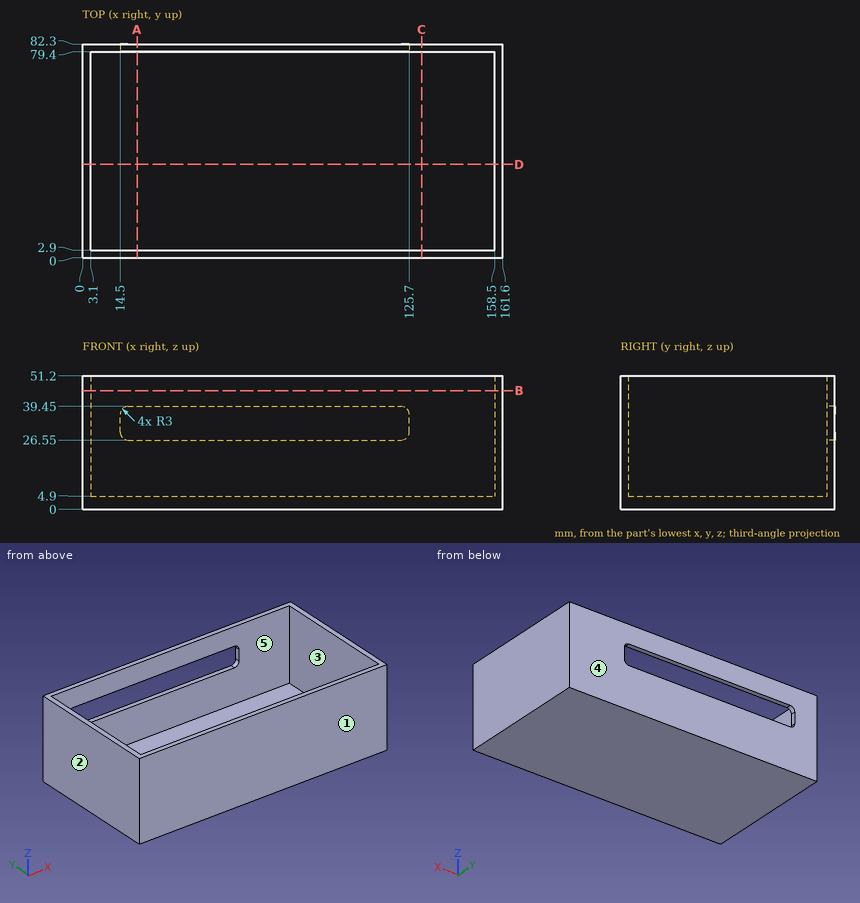
The figure shows three views and two pictorial views of one solid part (mm, origin at its lowest corner). Answer the questions. A direction names the side the tool comes from. Coordinates: 2 decimals unless noted, no trailing zeros. Order: outer loops, then holes, each group sorted by start corner. A loop starts at its lowest first (then second) coordinate and runs counter-clockwise, first axis right, second up.
Q1. Given P1, Ø8, axis at x = 45, y = 58.5, coming from the +Z side, flat-ended and moving along its own axis, determine where the tip first touches the part or whether it passes through.
Q2. A cutting plane is placed at A-A, the plane x = 21. Write down the section's boundary in (y, z).
Q3. A cutting plane is placed at C-C, the plane x = 130.5. Write down the section's boundary in (y, z), and give its area (3 significant figures).
Q4. A cutting plane is placed at D-D, the plane y = 36. Write down the section's boundary in (x, z), and give its area (3 significant figures).
Q5. For a pull along X with two mould halves and no side action, classify the marked faces 1, 2 and 3 as pulls with the +X half, pulls with the -X half, needs draft (parallel to the pull), parting line crosses it, or undercut.
Q6. Consider line 1 (Y direction, x = 85.5, z = 39.5); line 2 (X direction, y = 30.5, z = 28); line 3 (Z direction, x = 50, y = 66.5). Determine where each line is inside the solid, lowest interval first.
Q7. A cutting plane is placed at B-B, the plane z = 45.5. Write down the section's boundary in (x, y).
Q8. Which of the six approach directions +Z, -Z, +X, -X, +Y, -Y give full straight-line access (tool end or side, diameter ignored) to the marked faces 4 and 5?
Answers follow:
1. P1: stops at z = 4.9
2. outline: (0, 0) - (82.3, 0) - (82.3, 26.55) - (79.4, 26.55) - (79.4, 4.9) - (2.9, 4.9) - (2.9, 51.2) - (0, 51.2) - close; (79.4, 39.45) - (82.3, 39.45) - (82.3, 51.2) - (79.4, 51.2) - close
3. outline: (0, 0) - (82.3, 0) - (82.3, 51.2) - (79.4, 51.2) - (79.4, 4.9) - (2.9, 4.9) - (2.9, 51.2) - (0, 51.2) - close
3. area: 672 mm2
4. outline: (0, 0) - (161.6, 0) - (161.6, 51.2) - (158.5, 51.2) - (158.5, 4.9) - (3.1, 4.9) - (3.1, 51.2) - (0, 51.2) - close
4. area: 1,080 mm2
5. face 1: needs draft
5. face 2: pulls with the -X half
5. face 3: undercut
6. line 1: y = 0 to 2.9, 79.4 to 82.3
6. line 2: x = 0 to 3.1, 158.5 to 161.6
6. line 3: z = 0 to 4.9
7. outline: (0, 0) - (161.6, 0) - (161.6, 82.3) - (0, 82.3) - close; hole (3.1, 2.9) - (158.5, 2.9) - (158.5, 79.4) - (3.1, 79.4) - close
8. face 4: +Z, -Z, +X, -X, +Y
8. face 5: +Z
